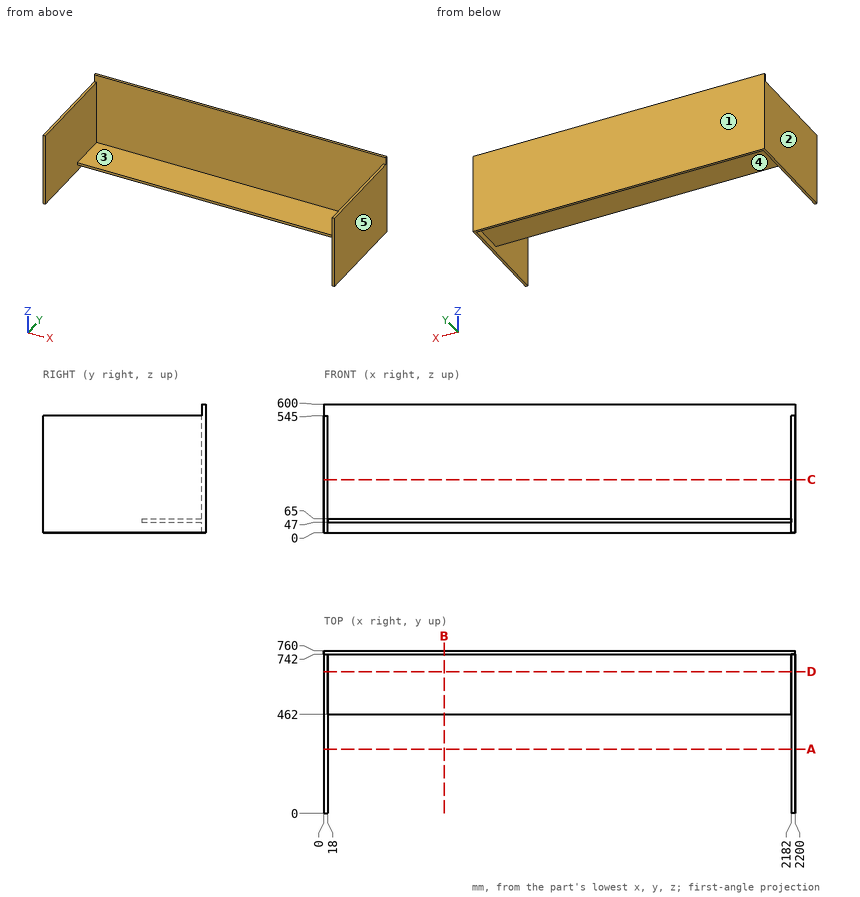
Job drawing, mm, ordinate dimensions from the low corner. One solid piece. A direction names the side the tool comes from. Round coordinates to 2 decimals unless told otherwise and drop trailing zeros. Order: outer loops, then holes, each group sorted by start corner. A loop starts at its lowest first (then second) coordinate and runs counter-clockwise, first axis right, second up. Notation, with made-up numbers: (-28.5, 29) -> (-17.5, 29) arc R3 cw to (-17.5, 34) -> close; hole circle Ø3 at (63.25, 47). An arc over 180 degrees is marked (long way). Answer in a Markdown table with one row per item.
1) Band-saw the part on A-A on y = 299.5. Give the cut face in (x, z), and give its area (3 significant figures).
Values:
| item | result |
|---|---|
| outline | (0, 0) -> (18, 0) -> (18, 545) -> (0, 545) -> close; (2182, 0) -> (2200, 0) -> (2200, 545) -> (2182, 545) -> close |
| area | 19,600 mm2 |
2) Band-saw the part on D-D on y = 661.5. Give the cut face in (x, z).
Values:
| item | result |
|---|---|
| outline | (0, 0) -> (18, 0) -> (18, 47) -> (2182, 47) -> (2182, 0) -> (2200, 0) -> (2200, 545) -> (2182, 545) -> (2182, 65) -> (18, 65) -> (18, 545) -> (0, 545) -> close |
3) Wall check: L1, parallel to X at y = 136, z = 429; L2, parallel to Y at x = 1295.5, z = 136; L3, parallel to Z at x = 279, y = 575. Give the ranges that are in metal, low to high.
Values:
| item | result |
|---|---|
| L1 | 0 to 18, 2182 to 2200 |
| L2 | 742 to 760 |
| L3 | 47 to 65 |
4) Band-saw the part on B-B on x = 562. Give the cut face in (y, z), and give its area (3 significant figures).
Values:
| item | result |
|---|---|
| outline | (462, 47) -> (742, 47) -> (742, 0) -> (760, 0) -> (760, 600) -> (742, 600) -> (742, 65) -> (462, 65) -> close |
| area | 15,800 mm2 |
5) Pin check, flat tips, straight feed: P1, Ø9, axis at x = 11.5, y = 441.5, coming from the +Z side; P2, Ø5.5, axis at x = 1448, z = 52.5, coming from the -Y side; P3, Ø6, axis at x = 1074.5, z = 459, coming from the -Y side. Stop position of each tip, or through.
Values:
| item | result |
|---|---|
| P1 | z = 545 |
| P2 | y = 462 |
| P3 | y = 742 |
6) Band-saw the part on C-C on z = 247. Give the cut face in (x, y).
Values:
| item | result |
|---|---|
| outline | (0, 0) -> (18, 0) -> (18, 742) -> (2182, 742) -> (2182, 0) -> (2200, 0) -> (2200, 760) -> (0, 760) -> close |
7) Which spindle directions (+Z, -Z, +X, -X, +Y, -Y) get a long thin tool onto all of the face, cutting with end or side? Do the marked faces 4 and 5. Say none if no direction does.
Values:
| item | result |
|---|---|
| face 4 | -Z, -Y |
| face 5 | +Z, -Z, +X, +Y, -Y |
8) Mould opens along X. For the marked faces 1, 2 and 3 say: released by +X, released by -X, zero draft, split by the parting line, or undercut.
Values:
| item | result |
|---|---|
| face 1 | zero draft |
| face 2 | released by -X |
| face 3 | undercut |
